```python
from build123d import *

# Parameters (mm, degrees)
F1_DEPTH = 914.4
F2_T     = -12.7
F3_R     = 12.7


with BuildPart() as f1:
    # F0 (on Front) → F1 (new body)
    with BuildSketch(Plane.XZ):
        Polygon((-863.6, 0), (0, 0), (0, 1016), (-215.9, 1016), (-215.9, 762), (-431.8, 762), (-431.8, 508), (-647.7, 508), (-647.7, 254), (-863.6, 254), align=None)
    extrude(amount=F1_DEPTH)

    # F2
    f2_openings = [f1.faces().sort_by_distance(p)[0] for p in [
        (-431.8, -457.2, 0),
    ]]
    offset(amount=F2_T, openings=f2_openings, kind=Kind.INTERSECTION)

    # F3
    f3_edges = [f1.edges().sort_by_distance(p)[0] for p in [
        (-647.7, -457.2, 254),
        (-431.8, -457.2, 508),
        (-215.9, -457.2, 762),
    ]]
    fillet(f3_edges, radius=F3_R)


solid = f1.part
```
The model under review builds one solid part; all positions refer to its coordinate system, in mm. A direction names the side the tool comes from. Give positions to 0.01 mm unless a question says otherwise; leave off trailing zeros. Order: outer loops, then holes, each group sorted by start corner. A loop starts at its lowest first (then second) coordinate and runs counter-clockwise, first axis right, second up. Notation, with made-up numbers: (-21.5, -6.75) - (-16.5, -6.75) arc R20 cw to (-16.5, 31.25) - close; hole circle Ø11 at (-2, -15). An arc over 180 degrees is marked (long way). Use CSV: the item, a comma, the result in double quotes. Start each with the question number.
Q1. The part is to be moulded in two halves that separate along X. For faces 1 (the flat face through (-342, -914.4, 402)), 2 (the flat face through (-635, -451, 370)), 3 (the flat face through (-647.7, -451, 389)), say which applies: +X half, -X half, draft (parallel to the pull), parting line (faces both ways), or undercut.
Q2. We need section A-A, the plane z = 212.5. Write out the cut boundary in (x, y).
Q3. To check wall thickness, follow line 1 along X through (y, z) = (-223, 282); line 2 along Y through (x, z) = (-52, 124); line 3 along X through (y, z) = (-528, 525). State the ranges of each line that lie inside material, in increasing order. Write a range as [from, to].
Q4. Clearance check with flat-ended pins moving along their axes: pin 1 Ø10 at (x, y) = (-261, -93) entering from +Z; pin 2 Ø4 at (x, z) = (-393, 451) entering from +Y; pin 3 Ø12 at (x, y) = (-741.5, -559.5) entering from +Z; pin 4 Ø6 at (x, y) = (-617, -166.5) entering from -Z. State where each tip first meets the part, or that it passes through.
Q5. We need section B-B, the plane x = -111. Write out the cut boundary in (y, z), and give its area (3 significant figures).
Q6. We need section C-C, the plane y = -476. Write out the cut boundary in (x, z).
Q7. We need section D-D, the plane z = 928. Write out the cut boundary in (x, y).
Q8. Tool access review of faces 4 (the flat face through (-215.9, -451, 897)), 5 (the flat face through (-863.6, -451, 129)), 6 (the flat face through (-107, -451, 1003.3)): name each direction out of +Z, -Z, +X, -X, +Y, -Y from which nothing blocks a thin tool from reaching the whole face with its end or side.
Outcome:
1,face 1,"draft"
1,face 2,"undercut"
1,face 3,"-X half"
2,outline,"(-863.6, -914.4) - (0, -914.4) - (0, 0) - (-863.6, 0) - close; hole (-850.9, -901.7) - (-12.7, -901.7) - (-12.7, -12.7) - (-850.9, -12.7) - close"
3,line 1,"x = [-647.7, -635], [-12.7, 0]"
3,line 2,"y = [-914.4, -901.7], [-12.7, 0]"
3,line 3,"x = [-431.8, -419.1], [-12.7, 0]"
4,pin 1,"stops at z = 762"
4,pin 2,"stops at y = 0"
4,pin 3,"stops at z = 254"
4,pin 4,"stops at z = 495.3"
5,outline,"(-914.4, 0) - (-901.7, 0) - (-901.7, 1003.3) - (-12.7, 1003.3) - (-12.7, 0) - (0, 0) - (0, 1016) - (-914.4, 1016) - close"
5,area,"37,100 mm^2"
6,outline,"(-863.6, 0) - (-850.9, 0) - (-850.9, 241.3) - (-635, 241.3) - (-635, 495.3) - (-419.1, 495.3) - (-419.1, 749.3) - (-203.2, 749.3) - (-203.2, 1003.3) - (-12.7, 1003.3) - (-12.7, 0) - (0, 0) - (0, 1016) - (-215.9, 1016) - (-215.9, 774.7) arc R12.7 cw to (-228.6, 762) - (-431.8, 762) - (-431.8, 520.7) arc R12.7 cw to (-444.5, 508) - (-647.7, 508) - (-647.7, 266.7) arc R12.7 cw to (-660.4, 254) - (-863.6, 254) - close"
7,outline,"(-215.9, -914.4) - (0, -914.4) - (0, 0) - (-215.9, 0) - close; hole (-203.2, -901.7) - (-12.7, -901.7) - (-12.7, -12.7) - (-203.2, -12.7) - close"
8,face 4,"+Z, -X, +Y, -Y"
8,face 5,"+Z, -Z, -X, +Y, -Y"
8,face 6,"-Z"
